Build history of the part. All positions in model axes, mm. Round coordinates to 2 decimals unless told otherwise and drop trailing zeros. Write each loop counter-clockwise with the first axis right and the second up, starting at its lowest first coordinate (ties: lowest second). Pieces come first, ordered by that corner, then holes. Notation, with made-up numbers: M 16.5,-30.5 L 54.5,-30.5 A19 ccw 54.5,5.5 Z; hole C -32.5,-32 d11. An arc over 180 degrees is marked long. Write item = value, one per line. Start each with the question number.
Q1. Band-saw the part on C-C on x = 4. Write the cut outline in (y, z) (3 decimals).
Q2. Band-saw the part on B-B on z = 0. Write the cut outline in (x, y) (3 decimals).
Q3. Drop flat-ended pins along their axis: P1, Ø0.8, axis at y = 2, z = -9, coming from the +X side; P2, Ø0.5, axis at x = 42.5, y = 2, coming from the -Z side; P3, Ø6, axis at x = 2, z = 8, coming from the -Y side. Give the stop position or say it passes through.
Q4. Probe L1, parallel to Z at x = -40, y = 1.15 (3 decimals); L2, parallel to Y at x = 34, z = -12; L3, parallel to X at y = 0.65, z = 10.5. List the from-to ranges inside material, lowest first.
Q5. Band-saw the part on A-A on x = -21. Write the cut outline in (y, z) (3 decimals).
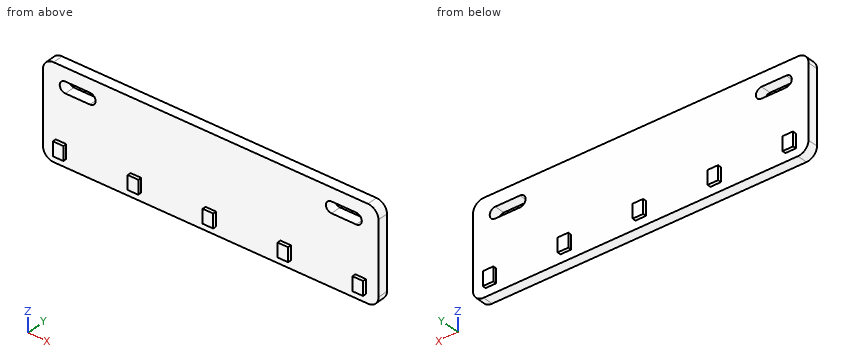
```python
from build123d import *

# Parameters (mm, degrees)
SKETCH_1_W                 = 95.25
SKETCH_1_H                 = 26.67
EXTRUDE_1_DEPTH            = 1.5
FILLET_1_R                 = 3
SKETCH_2_W                 = 3
SKETCH_2_H                 = 4
EXTRUDE_2_DEPTH            = 2.5
PATTERN_LINEAR_1_COUNT     = 3
PATTERN_LINEAR_1_PITCH     = 21.27
PATTERN_LINEAR_1_COL_COUNT = 3
PATTERN_LINEAR_1_COL_PITCH = 21.27


with BuildPart() as part:
    # 草图1 → 凸台-拉伸1 (new, symmetric)
    with BuildSketch(Plane(origin=(0, 0, 0), x_dir=(1, 0, 0), z_dir=(0, 1, 0))):
        Rectangle(SKETCH_1_W, SKETCH_1_H)
        with BuildLine():
            Line((34.29, -6.41), (41.29, -6.41))
            ThreePointArc((41.29, -6.41), (42.88, -8), (41.29, -9.59))
            Line((41.29, -9.59), (34.29, -9.59))
            ThreePointArc((34.29, -9.59), (32.7, -8), (34.29, -6.41))
        make_face(mode=Mode.SUBTRACT)
        with BuildLine():
            Line((-34.29, -6.41), (-41.29, -6.41))
            ThreePointArc((-41.29, -6.41), (-42.88, -8), (-41.29, -9.59))
            Line((-41.29, -9.59), (-34.29, -9.59))
            ThreePointArc((-34.29, -9.59), (-32.7, -8), (-34.29, -6.41))
        make_face(mode=Mode.SUBTRACT)
    extrude(amount=EXTRUDE_1_DEPTH, both=True)

    # 圆角1
    fillet_1_edges = [part.edges().sort_by_distance(p)[0] for p in [
        (47.625, 0, 13.335),
        (-47.625, 0, 13.335),
        (-47.625, 0, -13.335),
        (47.625, 0, -13.335),
    ]]
    fillet(fillet_1_edges, radius=FILLET_1_R)

    # 草图2 → 凸台-拉伸2 (add, symmetric)
    with BuildSketch(Plane(origin=(0, 0, 0), x_dir=(1, 0, 0), z_dir=(0, 1, 0))):
        with Locations((0, 9)):
            Rectangle(SKETCH_2_W, SKETCH_2_H)
    extrude_2 = extrude(amount=EXTRUDE_2_DEPTH, both=True)

    # 阵列(线性)1: 凸台-拉伸2 ×3
    with Locations(*[(i * PATTERN_LINEAR_1_PITCH, 0, 0) for i in range(1, PATTERN_LINEAR_1_COUNT)]):
        add(extrude_2)

    # 阵列(线性)1 col: 凸台-拉伸2 ×3
    with Locations(*[(-i * PATTERN_LINEAR_1_COL_PITCH, 0, 0) for i in range(1, PATTERN_LINEAR_1_COL_COUNT)]):
        add(extrude_2)


solid = part.part
```
Conclusion:
q1.outline = M -1.5,-13.335 L 1.5,-13.335 L 1.5,13.335 L -1.5,13.335 Z
q2.outline = M -47.625,-1.5 L 47.625,-1.5 L 47.625,1.5 L -47.625,1.5 Z
q3.P1 = 44.04
q3.P2 = -11
q3.P3 = -1.5
q4.L1 = -13.335 to 6.41, 9.59 to 13.335
q4.L2 = -1.5 to 1.5
q4.L3 = -47.62 to 47.62
q5.outline = M -2.5,-11 L -1.5,-11 L -1.5,-13.335 L 1.5,-13.335 L 1.5,-11 L 2.5,-11 L 2.5,-7 L 1.5,-7 L 1.5,13.335 L -1.5,13.335 L -1.5,-7 L -2.5,-7 Z
